Can you work these out from the model? Positions are in its coordinate system, mm. A direction names the side the tool comes from. Coordinates: 2 decimals unless noted, no trailing zeros. Order: outer loops, then holes, each group sorted by start corner. A loop starts at its lowest first (then second) coordinate and runs counter-clockwise, first axis right, second up. Notation, with made-up numbers: (11, -3.75) -> (26, -3.75) arc R22 cw to (26, 9.25) -> close; hole circle Ø4 at (-23, -8.5). An arc over 180 degrees is marked (long way). Answer in a Markdown table with one row per item. Add a question column.
1. We'd pull the mould along Z, two halves only. Please class faces 1 (the face through (18.75, 2, 14)), 2 (the face through (-28.4, 2.03, -0.09)), 3 (the face through (0, 2, 18.75)): pulls with the +Z half, pulls with the -Z half, needs draft (parallel to the pull), parting line crosses it, or undercut.
2. Imagine slicing it at C-C on y = 2.1. State how many separate pieces and enclosed holes the cut face has, plus the area to 3 significant figures.
3. Will these pins go through, and if not, where does the flat tip stop? pin 1 (2 mm diameter, centred on x = -19, y = 3, fed in from -Z); pin 2 (1.4 mm diameter, centred on y = 1.5, z = -14.5, fed in from +X); pin 3 (0.8 mm diameter, centred on y = 2, z = 14, fed in from -X); pin 4 (5.5 mm diameter, centred on x = -14.1, z = -14.1, fed in from -Y).
4. Imagine slicing it at D-D on x = -14.1. Write out the boundary of the cut face in (y, z).
5. Imagine slicing it at B-B on x = 26.25. Write out the boundary of the cut face in (y, z).
6. If I drill on line 1 along X through (y, z) = (1.5, 0); line 2 along Z through (x, y) = (14.1, 2.8), over which ranges is the centre line in solid material (lowest first)? Write a range as [from, to].
7. On a 3-axis mill with a long thin cutter (end or side, diameter ignored), from which of +Z, -Z, +X, -X, +Y, -Y can I reach the whole of each face in a straight line? I mean faces 4 (the face through (26, 2, 10)), 5 (the face through (26, 2, -10)), 6 (the face through (-18.75, 2, 14)). Say none if no direction works.
8. Imagine slicing it at A-A on z = 14.1. Write out the boundary of the cut face in (x, y), plus the area to 3 significant figures.
from build123d import *

# Parameters (mm, degrees)
SKETCH1_W               = 37.5
SKETCH1_H               = 37.5
BOSS_EXTRUDE1_DEPTH     = 4
FILLET1_R               = 3
SKETCH5_R               = 1.75
CUT_EXTRUDE2_DEPTH      = 1
CUT_EXTRUDE2_DEPTH_BACK = 5
SKETCH6_W               = 67.5
SKETCH6_H               = 20
BOSS_EXTRUDE2_DEPTH     = 4
FILLET2_R               = 3
SKETCH7_R               = 2.15
CUT_EXTRUDE3_DEPTH      = 1
CUT_EXTRUDE3_DEPTH_BACK = 5


with BuildPart() as part:
    # Sketch1 → Boss-Extrude1 (new body)
    with BuildSketch(Plane(origin=(0, 0, 0), x_dir=(1, 0, 0), z_dir=(0, 1, 0))):
        Rectangle(SKETCH1_W, SKETCH1_H)
    extrude(amount=BOSS_EXTRUDE1_DEPTH)

    # Fillet1
    fillet1_edges = [part.edges().sort_by_distance(p)[0] for p in [
        (18.75, 2, 18.75),
        (-18.75, 2, 18.75),
        (-18.75, 2, -18.75),
        (18.75, 2, -18.75),
    ]]
    fillet(fillet1_edges, radius=FILLET1_R)

    # Sketch5 → Cut-Extrude2 (cut, two sides)
    with BuildSketch(Plane(origin=(0, 4, 0), x_dir=(1, 0, 0), z_dir=(0, 1, 0))) as cut_extrude2_sk:
        with Locations((-14.1, 14.1)):
            Circle(SKETCH5_R)
        with Locations((14.1, 14.1)):
            Circle(SKETCH5_R)
        with Locations((14.1, -14.1)):
            Circle(SKETCH5_R)
        with Locations((-14.1, -14.1)):
            Circle(SKETCH5_R)
    extrude(amount=CUT_EXTRUDE2_DEPTH, mode=Mode.SUBTRACT)
    extrude(cut_extrude2_sk.sketch, amount=-CUT_EXTRUDE2_DEPTH_BACK, mode=Mode.SUBTRACT)

    # Sketch6 → Boss-Extrude2 (add)
    with BuildSketch(Plane.XZ):
        Rectangle(SKETCH6_W, SKETCH6_H)
    extrude(amount=-BOSS_EXTRUDE2_DEPTH)

    # Fillet2
    fillet2_edges = [part.edges().sort_by_distance(p)[0] for p in [
        (33.75, 2, -10),
        (18.75, 2, 10),
        (-18.75, 2, 10),
        (-33.75, 2, 10),
        (-33.75, 2, -10),
        (18.75, 2, -10),
        (-18.75, 2, -10),
        (33.75, 2, 10),
    ]]
    fillet(fillet2_edges, radius=FILLET2_R)

    # Sketch7 → Cut-Extrude3 (cut, two sides)
    with BuildSketch(Plane(origin=(0, 4, 0), x_dir=(1, 0, 0), z_dir=(0, 1, 0))) as cut_extrude3_sk:
        with Locations((-26.25, 0)):
            Circle(SKETCH7_R)
        with Locations((26.25, 0)):
            Circle(SKETCH7_R)
    extrude(amount=CUT_EXTRUDE3_DEPTH, mode=Mode.SUBTRACT)
    extrude(cut_extrude3_sk.sketch, amount=-CUT_EXTRUDE3_DEPTH_BACK, mode=Mode.SUBTRACT)


solid = part.part
Answers follow:
| question | item | result |
|---|---|---|
| 1 | face 1 | needs draft |
| 1 | face 2 | undercut |
| 1 | face 3 | pulls with the +Z half |
| 2 | separate pieces | 1 |
| 2 | enclosed holes | 6 |
| 2 | area | 1,930 mm² |
| 3 | pin 1 | stops at z = -17.73 |
| 3 | pin 2 | stops at x = 18.75 |
| 3 | pin 3 | stops at x = -18.75 |
| 3 | pin 4 | stops at y = 0 |
| 4 | outline | (0, -18.75) -> (4, -18.75) -> (4, -15.85) -> (0, -15.85) -> close; (0, -12.35) -> (4, -12.35) -> (4, 12.35) -> (0, 12.35) -> close; (0, 15.85) -> (4, 15.85) -> (4, 18.75) -> (0, 18.75) -> close |
| 5 | outline | (0, -10) -> (4, -10) -> (4, -2.15) -> (0, -2.15) -> close; (0, 2.15) -> (4, 2.15) -> (4, 10) -> (0, 10) -> close |
| 6 | line 1 | x = [-33.75, -28.4], [-24.1, 24.1], [28.4, 33.75] |
| 6 | line 2 | z = [-18.75, -15.85], [-12.35, 12.35], [15.85, 18.75] |
| 7 | face 4 | +Z, +X, +Y, -Y |
| 7 | face 5 | -Z, +X, +Y, -Y |
| 7 | face 6 | +Z, -X, +Y, -Y |
| 8 | outline | (-18.75, 0) -> (-15.85, 0) -> (-15.85, 4) -> (-18.75, 4) -> close; (-12.35, 0) -> (12.35, 0) -> (12.35, 4) -> (-12.35, 4) -> close; (15.85, 0) -> (18.75, 0) -> (18.75, 4) -> (15.85, 4) -> close |
| 8 | area | 122 mm² |
